from build123d import *

# Parameters (mm, degrees)
F0_W           = 20
F0_H           = 63
F1_DEPTH       = 8
F2_W           = 63
F2_H           = 55
F3_DEPTH       = 8
F5_D           = 4.572
F5_CBORE_D     = 7.62
F5_CBORE_DEPTH = 4.572
F6_W           = 47
F6_H           = 48
F7_DEPTH       = 28.001
F9_W           = 4
F9_H           = 51
F10_DEPTH      = 50
F12_DEPTH      = 5
F14_DEPTH      = 5
F16_DEPTH      = 25


# Not quite as in the source:
# - a feature names something its author has since deleted; it is built from what else it names


with BuildPart() as f1:
    # F0 (on Top) → F1 (new body)
    with BuildSketch(Plane.XY):
        Rectangle(F0_W, F0_H)
    extrude(amount=F1_DEPTH)

    # F2 (on face) → F3 (join)
    with BuildSketch(Plane.YZ.offset(10)):
        with Locations((0, 27.5)):
            Rectangle(F2_W, F2_H)
    extrude(amount=F3_DEPTH)

    # F5 (through all)
    with Locations(Plane.XY.offset(8)):
        with Locations((0, 0)):
            CounterBoreHole(F5_D / 2, F5_CBORE_D / 2, F5_CBORE_DEPTH)

    # F6 (on face) → F7 (cut, through all)
    with BuildSketch(Plane.YZ.offset(18)):
        with Locations((0, 31)):
            Rectangle(F6_W, F6_H)
    extrude(amount=-F7_DEPTH, mode=Mode.SUBTRACT)

    # F9 (on 3pt) → F10 (cut)
    with BuildSketch(Plane(origin=(0, 0, 55), x_dir=(1, 0, 0), z_dir=(0, 0, -1))):
        with Locations((14, 0)):
            Rectangle(F9_W, F9_H)
    extrude(amount=F10_DEPTH, mode=Mode.SUBTRACT)

    # F11 (on face) → F12 (join)
    with BuildSketch(Plane.XZ.offset(31.5)):
        Polygon((2, 8), (10, 8), (10, 24), align=None)
    extrude(amount=-F12_DEPTH)

    # F13 (on face) → F14 (join)
    with BuildSketch(Plane(origin=(0, 31.5, 0), x_dir=(-1, 0, 0), z_dir=(0, 1, 0))):
        Polygon((-10, 24), (-10, 8), (-2, 8), align=None)
    extrude(amount=-F14_DEPTH)

    # F15 (on face) → F16 (cut)
    with BuildSketch(Plane.XY.offset(8)):
        Polygon((-10, 11.5), (2, 31.5), (-10, 31.5), align=None)
        Polygon((-10, -11.5), (-10, -31.5), (2, -31.5), align=None)
    extrude(amount=-F16_DEPTH, mode=Mode.SUBTRACT)


solid = f1.part
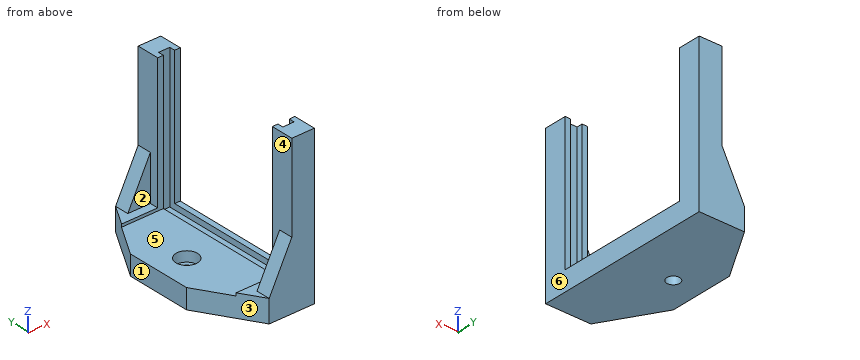
The listing builds one solid part. Answer for the finished solid, in the listing's coordinates (mm). Face numbers are marked on the shaded views. A direction names the side the tool comes from. Give positions to 0.01 mm unless a question says otherwise; leave off trailing zeros. Order: outer loops, then holes, each group sorted by start corner. A loop starts at its lowest first (then second) coordinate and runs counter-clockwise, first axis right, second up. Notation, with made-up numbers: (6, 52.25) -> (29, 52.25) arc R22 cw to (29, 63.25) -> close; hole circle Ø8 at (60.25, -13). An arc over 180 degrees is marked (long way). Put each result on its own line as item: value.
Item 1: Given P1, Ø2, axis at x = 14, y = -9.5, coming from the +Z side; P2, Ø10, axis at x = 2, y = 8.5, coming from the -Z side; P3, Ø6.5, axis at y = -29.5, z = 27, coming from the -X side (3 decimals); P4, Ø9, axis at y = 28, z = 37.5, coming from the -X side, each flat-ended and moving along its own axis, determine where each tip first touches the part or whether it passes through.
Established:
P1: stops at z = 5
P2: stops at z = 0
P3: stops at x = 9.875
P4: stops at x = 10
Item 2: Straight lines are drawn through the part: line 1 (Y direction, x = 11, z = 22); line 2 (Y direction, x = 13, z = 32.5); line 3 (Z direction, x = 6.25, y = -25.5). For each, find the intervals that lie inside material, in ascending order.
Established:
line 1: y = -31.5 to -23.5, 23.5 to 31.5
line 2: y = -31.5 to -25.5, 25.5 to 31.5
line 3: z = 0 to 8
Item 3: A cutting plane is placed at A-A on z = 17.5. Give the vertices of the cut face in (x, y), plus the area to 4 significant figures.
Established:
outline: (6.75, -31.5) -> (18, -31.5) -> (18, -23.5) -> (16, -23.5) -> (16, -25.5) -> (12, -25.5) -> (12, -23.5) -> (10, -23.5) -> (10, -26.5) -> (6.75, -26.5) -> close; (6.75, 26.5) -> (10, 26.5) -> (10, 23.5) -> (12, 23.5) -> (12, 25.5) -> (16, 25.5) -> (16, 23.5) -> (18, 23.5) -> (18, 31.5) -> (6.75, 31.5) -> close
area: 144.5 mm^2
Item 4: A cutting plane is placed at B-B on y = 0. Give the vertices of the cut face in (x, z), plus the area to 3 significant figures.
Established:
outline: (-10, 0) -> (-2.29, 0) -> (-2.29, 3.43) -> (-3.81, 3.43) -> (-3.81, 7) -> (-10, 7) -> close; (2.29, 0) -> (18, 0) -> (18, 7) -> (16, 7) -> (16, 5) -> (12, 5) -> (12, 7) -> (3.81, 7) -> (3.81, 3.43) -> (2.29, 3.43) -> close
area: 145 mm^2
Item 5: For the marked faces 4, 5 and 6, determine the directions among +Z, -Z, +X, -X, +Y, -Y from which every point of the face is accessible in a straight line to the end or side of a thin tool.
Established:
face 4: +Z, -X
face 5: +Z, +X, -X
face 6: +Z, -Z, +X, +Y, -Y
Item 6: A cutting plane is placed at C-C on x = 0. Give the vertices of the cut face in (y, z).
Established:
outline: (-28.17, 0) -> (-2.29, 0) -> (-2.29, 3.43) -> (-3.81, 3.43) -> (-3.81, 7) -> (-23.5, 7) -> (-23.5, 8) -> (-28.17, 8) -> close; (2.29, 0) -> (28.17, 0) -> (28.17, 8) -> (23.5, 8) -> (23.5, 7) -> (3.81, 7) -> (3.81, 3.43) -> (2.29, 3.43) -> close
Item 7: A cutting plane is placed at D-D on y = 15. Give the vertices of the cut face in (x, z).
Established:
outline: (-7.9, 0) -> (18, 0) -> (18, 7) -> (16, 7) -> (16, 5) -> (12, 5) -> (12, 7) -> (-7.9, 7) -> close
Item 8: For a pull along Y with two mould halves and no side action, classify the marked faces 1, 2 and 3 as released by +Y, released by -Y, zero draft, split by the parting line, or undercut.
Established:
face 1: zero draft
face 2: undercut
face 3: released by -Y
